```python
from build123d import *

# Parameters (mm, degrees)
SKETCH_2_W          = 57
SKETCH_2_H          = 40.4
EXTRUDE_1_DEPTH     = 1.5
SKETCH_4_R          = 3
SKETCH_4_R_2        = 1.5
EXTRUDE_3_DEPTH     = 16
SKETCH_5_W          = 57
SKETCH_5_H          = 4
CUT_EXTRUDE_1_DEPTH = 2.5
SKETCH_6_W          = 1
SKETCH_6_H          = 32.4
EXTRUDE_4_DEPTH     = 1.5


with BuildPart() as part:
    # 草图2 → 凸台-拉伸1 (new body)
    with BuildSketch(Plane(origin=(0, 0, 0), x_dir=(1, 0, 0), z_dir=(0, 1, 0))):
        with Locations((3.861898857, -4.534326193)):
            Rectangle(SKETCH_2_W, SKETCH_2_H)
    extrude(amount=EXTRUDE_1_DEPTH)

    # 草图4 → 凸台-拉伸3 (add)
    with BuildSketch(Plane(origin=(0, 1.5, 0), x_dir=(1, 0, 0), z_dir=(0, 1, 0))):
        with Locations((-22.099370277, 7.765673807)):
            Circle(SKETCH_4_R)
        with Locations((-22.099370277, 7.765673807)):
            Circle(SKETCH_4_R_2, mode=Mode.SUBTRACT)
        with Locations((-22.138101143, -16.834326193)):
            Circle(SKETCH_4_R)
        with Locations((-22.138101143, -16.834326193)):
            Circle(SKETCH_4_R_2, mode=Mode.SUBTRACT)
        with Locations((29.861898857, -16.834326193)):
            Circle(SKETCH_4_R)
        with Locations((29.861898857, -16.834326193)):
            Circle(SKETCH_4_R_2, mode=Mode.SUBTRACT)
        with Locations((29.861898857, 7.765673807)):
            Circle(SKETCH_4_R)
        with Locations((29.861898857, 7.765673807)):
            Circle(SKETCH_4_R_2, mode=Mode.SUBTRACT)
    extrude(amount=EXTRUDE_3_DEPTH)

    # 草图5 → 切除-拉伸1 (cut, through all)
    with BuildSketch(Plane(origin=(0, 1.5, 0), x_dir=(1, 0, 0), z_dir=(0, 1, 0))):
        with Locations((3.861898857, 13.665673807)):
            Rectangle(SKETCH_5_W, SKETCH_5_H)
        with Locations((3.861898857, -22.734326193)):
            Rectangle(SKETCH_5_W, SKETCH_5_H)
    extrude(amount=-CUT_EXTRUDE_1_DEPTH, mode=Mode.SUBTRACT)

    # 草图6 → 凸台-拉伸4 (add)
    with BuildSketch(Plane(origin=(0, 1.5, 0), x_dir=(1, 0, 0), z_dir=(0, 1, 0))):
        with Locations((-25.138101143, -4.534326193)):
            Rectangle(SKETCH_6_W, SKETCH_6_H)
        with Locations((32.861898857, -4.534326193)):
            Rectangle(SKETCH_6_W, SKETCH_6_H)
    extrude(amount=-EXTRUDE_4_DEPTH)


solid = part.part
```
Verification items for the finished model (mm, model axes). A direction names the side the tool comes from. Give positions to 0.01 mm unless a question says otherwise; leave off trailing zeros. Order: outer loops, then holes, each group sorted by start corner. A loop starts at its lowest first (then second) coordinate and runs counter-clockwise, first axis right, second up. Notation, with made-up numbers: (52.5, 66.5) - (108.5, 66.5) arc R25 cw to (108.5, 103.5) - close; hole circle Ø10 at (69.5, -5.5). An arc over 180 degrees is marked (long way). Answer as CSV lines item,"result". Start each with the question number.
Item 1: Mould release check, pull along Z, two halves, no side actions. Record for faces 3 (the face through (32.723, 9.388, -8.667)), 4 (the face through (-23.637, 9.388, 16.768)), 5 (the face through (3, 1, 20.734)), 6 (the face through (28, 17.5, -7)): released by +Z, released by -Z, zero draft, split by the parting line, or undercut.
Item 2: Section check C-C, the plane z = 16. Record the boundary of the cut face in (x, y).
Item 3: Material ranges on L1, parallel to Z at x = 28.5, y = 10; L2, parallel to X at y = 12.5, z = 18; L3, parallel to Y at x = 20.5, z = -2, recorded low to high.
Item 4: Section check B-B, the plane x = -22. Record the boundary of the cut face in (y, z), plus the area to 3 significant figures.
Item 5: Section check D-D, the plane z = -10. Record the boundary of the cut face in (x, y).
Item 6: Gauge pin test, flat ends, axial feed: pin 1 (0.9 mm diameter, centred on x = 30.5, z = -7.5, fed in from +Y); pin 2 (6 mm diameter, centred on x = -14, y = 11, fed in from +Z); pin 3 (2 mm diameter, centred on x = 27, y = 3, fed in from -Z). Record the tip position at first contact, or that the pin passes through.
Item 7: Access from +Z, -Z, +X, -X, +Y, -Y to the whole of each face (thin tool, end or side, straight path). Record for faces 1 (the face through (-24, 17.5, 17)), 2 (the face through (30, 1.5, 17)).
Item 8: Section check A-A, the plane y = 14.75. Record the boundary of the cut face in (x, z).
Filled in:
1,face 3,"undercut"
1,face 4,"undercut"
1,face 5,"released by +Z"
1,face 6,"zero draft"
2,outline,"(-25.64, 0) - (33.36, 0) - (33.36, 1.5) - (32.74, 1.5) - (32.74, 17.5) - (31.11, 17.5) - (31.11, 1.5) - (28.62, 1.5) - (28.62, 17.5) - (26.98, 17.5) - (26.98, 1.5) - (-19.26, 1.5) - (-19.26, 17.5) - (-20.89, 17.5) - (-20.89, 1.5) - (-23.38, 1.5) - (-23.38, 17.5) - (-25.02, 17.5) - (-25.02, 1.5) - (-25.64, 1.5) - close"
3,L1,"-10.44 to -8.39, -7.14 to -5.09, 14.16 to 16.21, 17.46 to 19.51"
3,L2,"-24.9 to -23.08, -21.19 to -19.37, 27.1 to 28.92, 30.81 to 32.63"
3,L3,"0 to 1.5"
4,outline,"(0, -11.67) - (1.5, -11.67) - (1.5, -10.76) - (17.5, -10.76) - (17.5, -9.26) - (1.5, -9.26) - (1.5, -6.27) - (17.5, -6.27) - (17.5, -4.77) - (1.5, -4.77) - (1.5, 13.84) - (17.5, 13.84) - (17.5, 15.34) - (1.5, 15.34) - (1.5, 18.33) - (17.5, 18.33) - (17.5, 19.83) - (1.5, 19.83) - (1.5, 20.73) - (0, 20.73) - close"
4,area,"145 mm^2"
5,outline,"(-25.64, 0) - (33.36, 0) - (33.36, 1.5) - (31.86, 1.5) - (31.86, 17.5) - (27.86, 17.5) - (27.86, 1.5) - (-20.1, 1.5) - (-20.1, 17.5) - (-24.1, 17.5) - (-24.1, 1.5) - (-25.64, 1.5) - close"
6,pin 1,"y = 1.5"
6,pin 2,"through"
6,pin 3,"z = -10.12"
7,face 1,"+Z, -Z, +X, -X, +Y"
7,face 2,"+Y"
8,outline,"circle Ø6 at (-22.14, 16.83); circle Ø6 at (-22.1, -7.77); circle Ø6 at (29.86, -7.77); circle Ø6 at (29.86, 16.83); hole circle Ø3 at (-22.14, 16.83); hole circle Ø3 at (-22.1, -7.77); hole circle Ø3 at (29.86, -7.77); hole circle Ø3 at (29.86, 16.83)"
